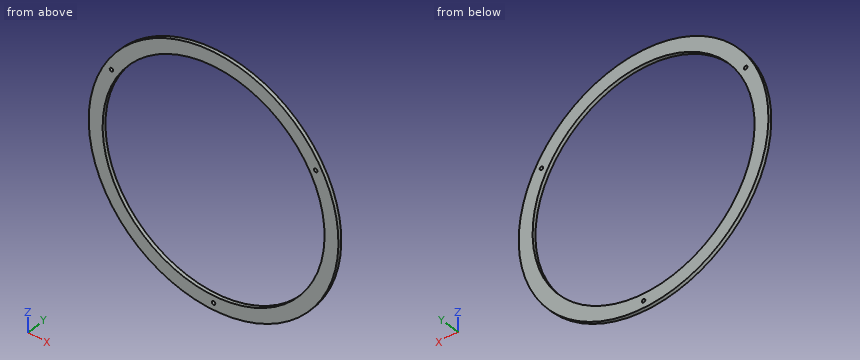
```python
from build123d import *

# Parameters (mm, degrees)
SKETCH1_R               = 228.6
BOSS_EXTRUDE1_DEPTH     = 6.35
CUT_EXTRUDE1_DEPTH      = 324.351577234
CUT_EXTRUDE1_DEPTH_BACK = 324.351577234
SKETCH2_R               = 3.175
CUT_EXTRUDE2_DEPTH      = 324.351577234
CUT_EXTRUDE2_DEPTH_BACK = 324.351577234
SKETCH3_R               = 203.2


with BuildPart() as part:
    # Sketch1 → Boss-Extrude1 (new body)
    with BuildSketch(Plane(origin=(0, 0, 0), x_dir=(1, 0, 0), z_dir=(0, 1, 0))):
        with Locations(Location((0, 0, 0), (0, 0, 270))):
            Circle(SKETCH1_R)
    extrude(amount=BOSS_EXTRUDE1_DEPTH)

    # Sketch2 → Cut-Extrude1 (cut, two sides: drawn at the far end of the back side and taken through both)
    with BuildSketch(Plane(origin=(0, 6.35, 0), x_dir=(1, 0, 0), z_dir=(0, 1, 0)).offset(-CUT_EXTRUDE1_DEPTH_BACK)):
        with Locations(Location((0, 215.9, 0), (0, 0, 270))):
            Circle(SKETCH2_R)
        with Locations(Location((-186.974884677, -107.95, 0), (0, 0, 270))):
            Circle(SKETCH2_R)
        with Locations(Location((186.974884677, -107.95, 0), (0, 0, 270))):
            Circle(SKETCH2_R)
    extrude(amount=CUT_EXTRUDE1_DEPTH + CUT_EXTRUDE1_DEPTH_BACK, mode=Mode.SUBTRACT)

    # Sketch3 → Cut-Extrude2 (cut, two sides: drawn at the far end of the back side and taken through both)
    with BuildSketch(Plane(origin=(0, 6.35, 0), x_dir=(1, 0, 0), z_dir=(0, 1, 0)).offset(-CUT_EXTRUDE2_DEPTH_BACK)):
        with Locations(Location((0, 0, 0), (0, 0, 270))):
            Circle(SKETCH3_R)
    extrude(amount=CUT_EXTRUDE2_DEPTH + CUT_EXTRUDE2_DEPTH_BACK, mode=Mode.SUBTRACT)


solid = part.part
```
For this review, take the finished solid that the model builds, in its own axes (mm). Round coordinates to 2 decimals unless told otherwise and drop trailing zeros. Write each loop counter-clockwise with the first axis right and the second up, starting at its lowest first coordinate (ties: lowest second). Pieces come first, ordered by that corner, then holes. Notation, with made-up numbers: (35, -23) - (75, -23) arc R25 cw to (75, -9) - close; hole circle Ø2 at (-1.5, -35.5). An arc over 180 degrees is marked (long way). Use CSV: the item, a comma, the result in double quotes.
1) Add section A-A on z = 0. Write out the cut boundary in (x, y).
Conclusion:
outline,"(-228.6, 0) - (-203.2, 0) - (-203.2, 6.35) - (-228.6, 6.35) - close; (203.2, 0) - (228.6, 0) - (228.6, 6.35) - (203.2, 6.35) - close"
2) Clearance check with flat-ended pins moving along their axes: pin 1 Ø3 at (x, y) = (-121, 5.5) entering from +Z; pin 2 Ø5.5 at (x, z) = (-186.97, 107.95) entering from -Y; pin 3 Ø1 at (y, z) = (2, -181) entering from +X; pin 4 Ø1 at (x, y) = (65, 2) entering from -Z. State where each tip first meets the part, or that it passes through.
Conclusion:
pin 1,"stops at z = 194.88"
pin 2,"passes through"
pin 3,"stops at x = 140.28"
pin 4,"stops at z = -219.31"
3) Add section C-C on y = 5.25. Write out the cut boundary in (x, z) (3 decimals).
Conclusion:
outline,"circle Ø457.2 at (0, 0); hole circle Ø406.4 at (0, 0); hole circle Ø6.35 at (-186.975, 107.95); hole circle Ø6.35 at (0, -215.9); hole circle Ø6.35 at (186.975, 107.95)"
4) Add section B-B on x = 78. Write out the cut boundary in (y, z), and give its area (3 significant figures).
Conclusion:
outline,"(0, -214.88) - (6.35, -214.88) - (6.35, -187.63) - (0, -187.63) - close; (0, 187.63) - (6.35, 187.63) - (6.35, 214.88) - (0, 214.88) - close"
area,"346 mm^2"
5) Wall thickness on line 1 along X through (y, z) = (2.5, 6.5); line 2 along X through (y, z) = (3, 0); line 3 along Z through (x, y) = (-5.5, 4): over which ranges is each line inside the solid? List them lowest first. Write a range as from..to.
Conclusion:
line 1,"x = -228.51..-203.1, 203.1..228.51"
line 2,"x = -228.6..-203.2, 203.2..228.6"
line 3,"z = -228.53..-203.13, 203.13..228.53"
